Check sheet for the drawn part. Datum: minimum x, y, z corner. Units: mm. A direction names the side the tool comes from. Give positions to 0.01 mm unless a question says otherwise; leave off trailing zeros. Loops run counter-clockwise (first coordinate to the right, second up) from the corner with the lowest first, then second, coordinate; pieces in that order, holes last.
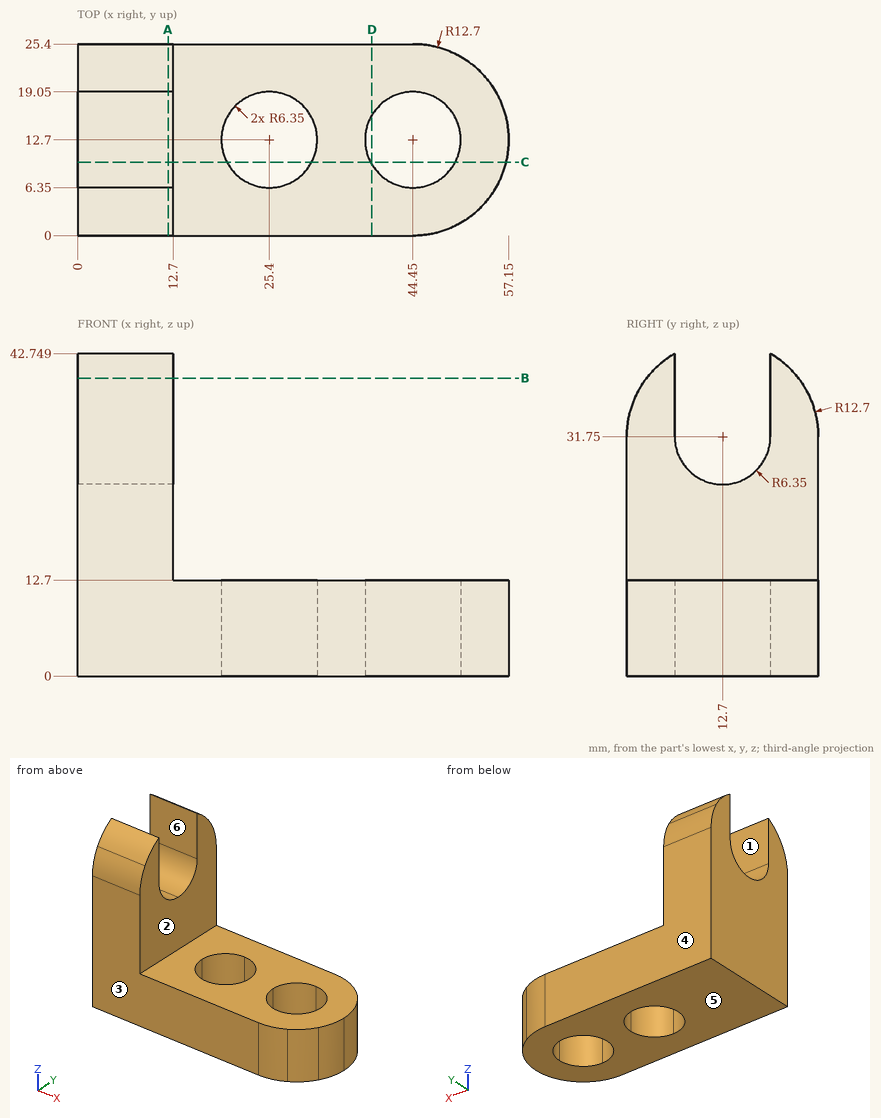
1) Sectioned sample at B-B on z = 39.5. Enter the section's corners in (x, y).
2) Scan lines: line 1 along Z through (x, y) = (19, 16.5); line 2 along X through (y, z) = (8, 6). Record each from-to range of solid material in increasing order.
3) Sectioned sample at D-D on x = 39. Enter the section's corners in (y, z), plus the area to 3 significant figures.
4) Sectioned sample at A-A on x = 12. Enter the section's corners in (y, z).
5) Sectioned sample at C-C on y = 9.75. Enter the section's corners in (x, z).
6) Depth check by flat-ended pin: P1, Ø1, axis at y = 10.5, z = 27.5, coming from the +X side; P2, Ø3.5, axis at x = 4, z = 39.5, coming from the -Y side; P3, Ø12, axis at x = 24.5, y = 2.5, coming from the +Z side. Enter the tip coordinate at first touch or a pass-through.
7) Tool access check on the marked faces 1, 2 and 3. Record the directions out of +Z, -Z, +X, -X, +Y, -Y that give a thin tool (end or side, any length) a straight path to the whole face; none if there is none.
8) Mould release check, pull along Y, two halves, no side actions. Record for the marked faces 4, 5 and 6: +Y half, -Y half, draft (parallel to the pull), parting line (faces both ways), or undercut.
Determined:
1. outline: (0, 2.64) - (12.7, 2.64) - (12.7, 6.35) - (0, 6.35) - close; (0, 19.05) - (12.7, 19.05) - (12.7, 22.76) - (0, 22.76) - close
2. line 1: z = 0 to 12.7
2. line 2: x = 0 to 21.13, 29.67 to 40.18, 48.72 to 56.25
3. outline: (0, 0) - (9.44, 0) - (9.44, 12.7) - (0, 12.7) - close; (15.96, 0) - (25.4, 0) - (25.4, 12.7) - (15.96, 12.7) - close
3. area: 240 mm2
4. outline: (0, 0) - (25.4, 0) - (25.4, 31.75) arc R12.7 ccw to (19.05, 42.75) - (19.05, 31.75) arc R6.35 cw to (6.35, 31.75) - (6.35, 42.75) arc R12.7 ccw to (0, 31.75) - close
5. outline: (0, 0) - (19.78, 0) - (19.78, 12.7) - (12.7, 12.7) - (12.7, 26.13) - (0, 26.13) - close; (31.02, 0) - (38.83, 0) - (38.83, 12.7) - (31.02, 12.7) - close; (50.07, 0) - (56.8, 0) - (56.8, 12.7) - (50.07, 12.7) - close
6. P1: passes through
6. P2: stops at y = 1.51
6. P3: stops at z = 12.7
7. face 1: +Z, +X, -X
7. face 2: +Z, +X, +Y, -Y
7. face 3: +Z, -Z, +X, -X, -Y
8. face 4: +Y half
8. face 5: draft
8. face 6: undercut
